Part model, mm, in its own coordinate system. A direction names the side the tool comes from. Round coordinates to 2 decimals unless told otherwise and drop trailing zeros. Loops run counter-clockwise (first coordinate to the right, second up) from the corner with the lowest first, then second, coordinate; pieces in that order, holes last.
(1) Probe probe 1 along X at (y, z) = (45, -0.5); probe 2 along Y at (x, z) = (-45, -6.5); probe 3 along Y at (x, z) = (-67.5, -5.05). List the from-to ranges inside material, lowest first.
(2) Cut at A-A on y = 32.5. List the corners of the cut face in (x, z).
(3) Cut at D-D on z = -6.75. Count the separate pieces of the cut face and the enclosed holes in it, then the cut area to 3 significant figures.
(4) Tool access for faces 1 (the face through (-1, 1, 0)), 2 (the face through (83.31, 32.42, -3.94)), 3 (the face through (-68.58, -70.12, -5.54)): list every direction of +Z, -Z, +X, -X, +Y, -Y with a clear straight run to the whole face (end or side of a thin tool).
(5) Cut at B-B on x = 12.5. List the corners of the cut face in (y, z).
(6) Mould opens along Y. For faces 4 (the face through (87.5, -1, -4)), 5 (the face through (-1, 92.5, -4)), 6 (the face through (71.31, 2.58, -3.94)) say: +Y half, -Y half, draft (parallel to the pull), parting line (faces both ways), or undercut.
(7) Cut at C-C on y = -85.5. List the corners of the cut face in (x, z).
from build123d import *

# Parameters (mm, degrees)
F0_W           = 175
F0_H           = 185
F1_DEPTH       = 8
F2_R           = 3.25
F2_R_2         = 3.5
F2_R_3         = 10
F2_R_4         = 20
F3_DEPTH       = 25
F5_D           = 6
F5_DEPTH       = 15
F5_CBORE_D     = 10
F5_CBORE_DEPTH = 5


with BuildPart() as f1:
    # F0 (on Top) → F1 (new body)
    with BuildSketch(Plane.XY):
        Rectangle(F0_W, F0_H)
    extrude(amount=-F1_DEPTH)

    # F2 (on face) → F3 (cut)
    with BuildSketch(Plane.XY):
        with Locations((-80, 85.5)):
            Circle(F2_R)
        with Locations((-40, 85.5)):
            Circle(F2_R)
        with Locations((-40, 45.5)):
            Circle(F2_R)
        with Locations((-80, 45.5)):
            Circle(F2_R)
        with Locations((40, 85.5)):
            Circle(F2_R)
        with Locations((80, 85.5)):
            Circle(F2_R)
        with Locations((40, 45.5)):
            Circle(F2_R)
        with Locations((80, 45.5)):
            Circle(F2_R)
        with BuildLine():
            Line((77.31, 29), (79.81, 29))
            ThreePointArc((79.81, 29), (83.31, 32.5), (79.81, 36))
            Line((79.81, 36), (74.81, 36))
            ThreePointArc((74.81, 36), (71.31, 32.5), (74.81, 29))
            Line((74.81, 29), (77.31, 29))
        make_face()
        with BuildLine():
            ThreePointArc((79.81, -1), (83.31, 2.5), (79.81, 6))
            Line((79.81, 6), (74.81, 6))
            ThreePointArc((74.81, 6), (71.31, 2.5), (74.81, -1))
            Line((74.81, -1), (79.81, -1))
        make_face()
        with Locations((42, 0)):
            Circle(F2_R_2)
        with Locations((42, -27.5)):
            Circle(F2_R_3)
        with Locations((40, -45.5)):
            Circle(F2_R)
        with Locations((80, -85.5)):
            Circle(F2_R)
        with Locations((80, -45.5)):
            Circle(F2_R)
        with Locations((40, -85.5)):
            Circle(F2_R)
        with Locations((-40, -85.5)):
            Circle(F2_R)
        with Locations((-80, -85.5)):
            Circle(F2_R)
        with Locations((-80, -45.5)):
            Circle(F2_R)
        with Locations((-40, -45.5)):
            Circle(F2_R)
        with Locations((-42, -27.5)):
            Circle(F2_R_3)
        with Locations((-42, 0)):
            Circle(F2_R_2)
        with Locations((0, -42.5)):
            Circle(F2_R_4)
    extrude(amount=-F3_DEPTH, mode=Mode.SUBTRACT)

    # F5
    with Locations(Plane(origin=(0, 0, -8), x_dir=(1, 0, 0), z_dir=(0, 0, -1))):
        with Locations((-67.5, 75), (67.5, 75)):
            CounterBoreHole(F5_D / 2, F5_CBORE_D / 2, F5_CBORE_DEPTH, depth=F5_DEPTH)


solid = f1.part
Final values:
1. probe 1: x = -87.5 to -83.21, -76.79 to -43.21, -36.79 to 36.79, 43.21 to 76.79, 83.21 to 87.5
1. probe 2: y = -92.5 to -37.04, -17.96 to -1.8, 1.8 to 92.5
1. probe 3: y = -92.5 to -80, -70 to 92.5
2. outline: (-87.5, -8) - (71.31, -8) - (71.31, 0) - (-87.5, 0) - close; (83.31, -8) - (87.5, -8) - (87.5, 0) - (83.31, 0) - close
3. separate pieces: 1
3. enclosed holes: 25
3. area: 29,600 mm2
4. face 1: +Z, +X, -X, +Y, -Y
4. face 2: +Z, -Z
4. face 3: -Z
5. outline: (-92.5, -8) - (-58.11, -8) - (-58.11, 0) - (-92.5, 0) - close; (-26.89, -8) - (92.5, -8) - (92.5, 0) - (-26.89, 0) - close
6. face 4: draft
6. face 5: +Y half
6. face 6: undercut
7. outline: (-87.5, -8) - (-83.25, -8) - (-83.25, 0) - (-87.5, 0) - close; (-76.75, -8) - (-43.25, -8) - (-43.25, 0) - (-76.75, 0) - close; (-36.75, -8) - (36.75, -8) - (36.75, 0) - (-36.75, 0) - close; (43.25, -8) - (76.75, -8) - (76.75, 0) - (43.25, 0) - close; (83.25, -8) - (87.5, -8) - (87.5, 0) - (83.25, 0) - close
